Input: part model. Units: mm. Frame: model coordinates. A direction names the side the tool comes from. Round coordinates to 2 decimals unless told otherwise and drop trailing zeros. Write each loop counter-clockwise with the first axis right and the second up, starting at its lowest first coordinate (ties: lowest second). Pieces come first, ordered by that corner, then holes. Notation, with made-up numbers: (24.5, 44) - (29.5, 44) arc R21 ccw to (29.5, 80) - close; hole circle Ø3 at (50.25, 62). An arc over 180 degrees is marked (long way). Use one line per item in the form item = value.
Autodesk Inventor part; units mm, degrees
ref_plane "YZ Plane" through (0, 0, 0) normal (1, 0, 0) x (0, 1, 0)
ref_plane "XZ Plane" through (0, 0, 0) normal (0, 1, 0) x (-1, 0, 0)
ref_plane "XY Plane" through (0, 0, 0) normal (0, 0, 1) x (1, 0, 0)
sketch "Sketch1" plane through (0, 0, 0) normal (0, 0, 1) x (1, 0, 0)
  line L0 (-13, 37.5) -> (13, 37.5)
  line L1 (13, 37.5) -> (13, -37.5)
  line L2 (13, -37.5) -> (-13, -37.5)
  line L3 (-13, -37.5) -> (-13, 37.5)
  point P0 (0, 0)
  point P1 (-13, 0)
  point P2 (0, 37.5)
  dimension "d0" = 26
  dimension "d2" = 75
extrude "Extrusion1" add sketch "Sketch1" along normal blind 6.477
sketch "Sketch2" plane through (0, 0, 6.477) normal (0, 0, 1) x (1, 0, 0)
  line L0 (13, 37.5) -> (-13, 37.5)
  line L1 (-5.3033, 35) -> (5.3033, 35)
  line L2 (5.3033, 35) -> (5.3033, 11)
  line L3 (5.3033, 11) -> (-5.3033, 11)
  line L4 (-5.3033, 11) -> (-5.3033, 35)
  circle A0 centre (0, 35) radius 7.5
  line L5 (0, 35) -> (5.3033, 29.6967)
  point P0 (0, 0)
  point P1 (0, 37.5)
  dimension "d7" = 15
  dimension "d5" = 35
  dimension "d6" = 45
  dimension "d8" = 24
extrude "Extrusion2" cut sketch "Sketch2" against normal through all contours A0 L2 L3 L4 | L4 L1 L5 A0 | L5 L1 L2
sketch "Sketch3" plane through (0, 0, 6.477) normal (0, 0, 1) x (1, 0, 0)
  line L0 (-5.3033, 11) -> (-5.3033, 35)
  line L1 (-5.3033, 35) -> (5.3033, 35)
  line L2 (-7.5, 28) -> (7.5, 28) construction
  line L3 (7.5, 28) -> (7.5, 18) construction
  line L4 (7.5, 18) -> (-7.5, 18) construction
  line L5 (-7.5, 18) -> (-7.5, 28) construction
  line L6 (-7.5, 28) -> (-9, 28)
  line L7 (-9, 28) -> (-9, 32)
  line L8 (-9, 32) -> (-7.5, 32)
  line L9 (-7.5, 32) -> (-7.5, 28)
  line L10 (7.5, 28) -> (9, 28)
  line L11 (9, 28) -> (9, 32)
  line L12 (9, 32) -> (7.5, 32)
  line L13 (7.5, 32) -> (7.5, 28)
  line L14 (7.5, 18) -> (9, 18)
  line L15 (9, 18) -> (9, 14)
  line L16 (9, 14) -> (7.5, 14)
  line L17 (7.5, 14) -> (7.5, 18)
  line L18 (-7.5, 18) -> (-9, 18)
  line L19 (-9, 18) -> (-9, 14)
  line L20 (-9, 14) -> (-7.5, 14)
  line L21 (-7.5, 14) -> (-7.5, 18)
  point P0 (0, 0)
  point P1 (0, 28)
  point P2 (0, 35)
  point P3 (-7.5, 23)
  point P4 (-5.3033, 23)
  point P5 (-7.5, 30)
  dimension "d11" = 4
  dimension "d13" = 1.5
  dimension "d14" = 15
  dimension "d15" = 5
extrude "Extrusion3" cut sketch "Sketch3" against normal through all
mirror "Mirror1" about plane through (0, 0, 0) normal (0, 1, 0) of "Extrusion3", "Extrusion2"
sketch "Sketch4" plane through (-5.3033, 35, 6.477) normal (0, -1, 0) x (1, 0, 0)
  line L0 (10.6066, -6.477) -> (0, -6.477)
  line L1 (10.6066, 0) -> (10.6066, -6.477)
  line L2 (0, 0) -> (10.6066, 0)
  line L3 (0, 0) -> (0, -6.477)
  arc A0 (0, 0) -> (10.6066, 0) centre (5.3033, 5.3033) ccw
  point P0 (5.3033, -6.477)
  dimension "d18" = 15
extrude "Extrusion4" add sketch "Sketch4" along normal up to surface (70 mm away) contours L0 L3 A0 L1
fillet "Fillet1" radius 5 4 edges at (13, -37.5, 3.2385) (13, 37.5, 3.2385) (-13, 37.5, 3.2385) (-13, -37.5, 3.2385)
properties part number "Y BEARING BLOCK"
(1) Cut plane C-C on x = 3.75. Output: boundary loops of the cut face in (y, z).
Derived:
outline = (-37.5, 0) - (37.5, 0) - (37.5, 6.48) - (35, 6.48) - (35, 5.29) - (11, 5.29) - (11, 6.48) - (-11, 6.48) - (-11, 5.29) - (-35, 5.29) - (-35, 6.48) - (-37.5, 6.48) - close
(2) Cut plane D-D on z = 1.25. Count the separate pieces of the cut face and the enclosed holes in it, then the cut area to 3 significant figures.
Derived:
separate_pieces = 1
enclosed_holes = 8
area = 1,880 mm^2
(3) Cut plane B-B on y = -25. Output: boundary loops of the cut face in (x, z).
Derived:
outline = (-13, 0) - (13, 0) - (13, 6.48) - (5.3, 6.48) arc R7.5 cw to (-5.3, 6.48) - (-13, 6.48) - close
(4) Access query for faces 5 (the face through (0, -37.5, 3)), 6 (the face through (7.5, 30, 3)). Directions: +Z, -Z, +X, -X, +Y, -Y. A direction counts if a zero-diameter tool reaches every point of the face in a straight line with its end or side. Return the directions, or none.
Derived:
face_5 = +Z, -Z, +X, -X, -Y
face_6 = +Z, -Z
(5) Cut plane A-A on y = -16. Output: boundary loops of the cut face in (x, z).
Derived:
outline = (-13, 0) - (-9, 0) - (-9, 6.48) - (-13, 6.48) - close; (-7.5, 0) - (7.5, 0) - (7.5, 6.48) - (5.3, 6.48) arc R7.5 cw to (-5.3, 6.48) - (-7.5, 6.48) - close; (9, 0) - (13, 0) - (13, 6.48) - (9, 6.48) - close
(6) Draft query along X for faces 1 (the face through (-9, 16, 3)), 2 (the face through (0, 37.5, 3)), 3 (the face through (-8, 14, 3)), 4 (the face through (-11.5, 36.07, 3.28)). Return one class per face: released by +X, released by -X, zero draft, split by the parting line, or undercut.
Derived:
face_1 = undercut
face_2 = zero draft
face_3 = undercut
face_4 = released by -X
(7) Material intervals for L1, parallel to Y at x = -3, z = 6; L2, parallel to Y at x = -8, z = 4.5; L3, parallel to Y at x = 8.75, z = 3.75, sorted ascending.
Derived:
L1 = -37.5 to -35, -11 to 11, 35 to 37.5
L2 = -37.5 to -32, -28 to -18, -14 to 14, 18 to 28, 32 to 37.5
L3 = -37.44 to -32, -28 to -18, -14 to 14, 18 to 28, 32 to 37.44
